For this review, take the finished solid that the model builds, in its own axes (mm). Round coordinates to 2 decimals unless told otherwise and drop trailing zeros. Loops run counter-clockwise (first coordinate to the right, second up) from the corner with the lowest first, then second, coordinate; pieces in that order, holes last. Notation, with made-up numbers: (72, 22) -> (90, 22) arc R36 cw to (90, 61) -> close; hole circle Ø11 at (60, -21). An arc over 180 degrees is marked (long way). Write each question's results on one line, items separated by ' | '.
```python
from build123d import *

# Parameters (mm, degrees)
ESQUISSE1_R             = 2.9
ESQUISSE1_R_2           = 0.5
BOSS_EXTRU_1_DEPTH      = 6
ESQUISSE2_R             = 4.232956527
ENL_V_MAT_EXTRU_1_DEPTH = 3


with BuildPart() as part:
    # Esquisse1 → Boss.-Extru.1 (new body)
    with BuildSketch(Plane.ZY.offset(-51.2)):
        with BuildLine():
            Line((-16.960725558, -57.422608764), (-46.752392225, -59.913913086))
            ThreePointArc((-46.752392225, -59.913913086), (-50.419058892, -63.9), (-46.752392225, -67.886086914))
            Line((-46.752392225, -67.886086914), (-16.960725558, -70.377391236))
            ThreePointArc((-16.960725558, -70.377391236), (-9.919058892, -63.9), (-16.960725558, -57.422608764))
        make_face()
        with Locations(Location((-16.419058892, -63.9, 0), (0, 0, 270))):
            Circle(ESQUISSE1_R, mode=Mode.SUBTRACT)
        with Locations(Location((-31.419058892, -63.9, 0), (0, 0, 270))):
            Circle(ESQUISSE1_R_2, mode=Mode.SUBTRACT)
        with Locations(Location((-44.419058892, -63.9, 0), (0, 0, 270))):
            Circle(ESQUISSE1_R_2, mode=Mode.SUBTRACT)
    extrude(amount=BOSS_EXTRU_1_DEPTH)

    # Esquisse2 → Enlèv. mat.-Extru.1 (cut)
    with BuildSketch(Plane(origin=(51.2, 0, 0), x_dir=(0, 0, -1), z_dir=(1, 0, 0))):
        with BuildLine():
            Line((16.960725558, -70.377391236), (46.752392225, -67.886086914))
            ThreePointArc((46.752392225, -67.886086914), (50.419058892, -63.9), (46.752392225, -59.913913086))
            Line((46.752392225, -59.913913086), (16.960725558, -57.422608764))
            ThreePointArc((16.960725558, -57.422608764), (9.919058892, -63.9), (16.960725558, -70.377391236))
        make_face()
        with Locations(Location((16.419058892, -63.9, 0), (0, 0, 90))):
            Circle(ESQUISSE2_R, mode=Mode.SUBTRACT)
    extrude(amount=-ENL_V_MAT_EXTRU_1_DEPTH, mode=Mode.SUBTRACT)


solid = part.part
```
1. Consider section D-D (z = -33.5). State the section outline as (x, y) points, plus the area to 3 significant figures.
Values found:
outline: (45.2, -68.99) -> (48.2, -68.99) -> (48.2, -58.81) -> (45.2, -58.81) -> close | area: 30.6 mm2
2. Consider section A-A (y = -63.9). State the section outline as (x, z) points.
Values found:
outline: (45.2, -50.42) -> (48.2, -50.42) -> (48.2, -44.92) -> (45.2, -44.92) -> close; (45.2, -43.92) -> (48.2, -43.92) -> (48.2, -31.92) -> (45.2, -31.92) -> close; (45.2, -30.92) -> (48.2, -30.92) -> (48.2, -20.65) -> (51.2, -20.65) -> (51.2, -19.32) -> (45.2, -19.32) -> close; (45.2, -13.52) -> (51.2, -13.52) -> (51.2, -12.19) -> (48.2, -12.19) -> (48.2, -9.92) -> (45.2, -9.92) -> close
3. Draft analysis for pull direction Z (two halves, no side actions). For faces 1 (the face through (48.242, -61.003, -16.292)), 2 (the face through (49.72, -68.13, -16.23)), 3 (the face through (51.2, -67, -17)), state which applies: released by +Z, released by -Z, zero draft, split by the parting line, or undercut.
Values found:
face 1: undercut | face 2: split by the parting line | face 3: zero draft
4. Consider section C-C (x = 47.5). State the section outline as (y, z) points.
Values found:
outline: (-70.38, -16.96) -> (-67.89, -46.75) arc R4 ccw to (-59.91, -46.75) -> (-57.42, -16.96) arc R6.5 ccw (long way) to start; hole circle Ø5.8 at (-63.9, -16.42); hole circle Ø1 at (-63.9, -44.42); hole circle Ø1 at (-63.9, -31.42)
5. For pin 1 (1 mm diameter, centred on x = 46.5, y = -61.5, fed in from -Z); pin 2 (1 mm diameter, centred on x = 50, y = -66.5, fed in from +Z); pin 3 (1 mm diameter, centred on y = -60.5, z = -40, fed in from +X); pin 4 (1 mm diameter, centred on x = 49.5, y = -59, fed in from +Z), all flat-tipped, find the tip position at first contact; note any pin that passes through.
Values found:
pin 1: stops at z = -49.94 | pin 2: stops at z = -12.74 | pin 3: stops at x = 48.2 | pin 4: passes through
6. To check wall thickness, follow probe 1 along Z at (x, y) = (47.05, -63.9); probe 2 along Z at (x, y) = (50.25, -64); probe 3 along X at (y, z) = (-62, -44.5). State the ranges of each line that lie inside material, in increasing order.
Values found:
probe 1: z = -50.42 to -44.92, -43.92 to -31.92, -30.92 to -19.32, -13.52 to -9.92 | probe 2: z = -20.65 to -19.32, -13.52 to -12.19 | probe 3: x = 45.2 to 48.2
7. Consider section B-B (z = -15.5). State the section outline as (x, y) points.
Values found:
outline: (45.2, -70.33) -> (48.2, -70.33) -> (48.2, -68.03) -> (51.2, -68.03) -> (51.2, -66.65) -> (45.2, -66.65) -> close; (45.2, -61.15) -> (51.2, -61.15) -> (51.2, -59.77) -> (48.2, -59.77) -> (48.2, -57.47) -> (45.2, -57.47) -> close
